Work out the finished part from the listing and answer in its coordinate system (mm). Round coordinates to 2 decimals unless told otherwise and drop trailing zeros. Write each loop counter-clockwise with the first axis right and the second up, starting at its lowest first coordinate (ties: lowest second). Pieces come first, ordered by that corner, then holes. Notation, with made-up numbers: (-0.75, 66) - (53.25, 66) arc R18 cw to (53.25, 97) - close; hole circle Ø5 at (0, -26.75). An arc over 180 degrees is marked (long way). Answer as a JSON object with one key per item and string values.
Autodesk Inventor part; units mm, degrees
ref_plane "YZ Plane" through (0, 0, 0) normal (1, 0, 0) x (0, 1, 0)
ref_plane "XZ Plane" through (0, 0, 0) normal (0, 1, 0) x (-1, 0, 0)
ref_plane "XY Plane" through (0, 0, 0) normal (0, 0, 1) x (1, 0, 0)
sketch "Sketch1" plane through (0, 0, 0) normal (0, 0, 1) x (1, 0, 0)
  line L0 (-262.5, 75) -> (262.5, 75)
  line L1 (262.5, 75) -> (262.5, 0)
  line L2 (262.5, 0) -> (-262.5, 0)
  line L3 (-262.5, 0) -> (-262.5, 75)
  line L4 (-262.5, 50) -> (-268.977, 50)
  line L5 (-268.977, 50) -> (-268.977, 25)
  line L6 (-268.977, 25) -> (-262.5, 25)
  line L7 (-262.5, 25) -> (-262.5, 50)
  line L8 (-212.5, 75) -> (-187.5, 75)
  line L9 (-187.5, 75) -> (-187.5, 81.477)
  line L10 (-187.5, 81.477) -> (-212.5, 81.477)
  line L11 (-212.5, 81.477) -> (-212.5, 75)
  line L12 (-12.5, 75) -> (12.5, 75)
  line L13 (12.5, 75) -> (12.5, 81.477)
  line L14 (12.5, 81.477) -> (-12.5, 81.477)
  line L15 (-12.5, 81.477) -> (-12.5, 75)
  point P0 (0, 0)
  point P1 (0, 0)
  point P2 (-268.977, 37.5)
  point P3 (-262.5, 37.5)
  point P4 (0, 81.477)
  point P5 (0, 75)
  dimension "d0" = 525
  dimension "d2" = 75
  dimension "d3" = 25
  dimension "d4" = 6.477
  dimension "d5" = 50
extrude "Extrusion1" add sketch "Sketch1" along normal blind 6.477
mirror "Mirror1" about plane through (0, 0, 0) normal (1, 0, 0) of "Extrusion1"
sketch "Sketch2" plane through (0, 0, 6.477) normal (0, 0, 1) x (1, 0, 0)
  line L0 (-187.5, 81.477) -> (-212.5, 81.477)
  line L1 (-262.5, 75) -> (-262.5, 50)
  line L2 (-268.977, 50) -> (-268.977, 25)
  line L3 (12.5, 81.477) -> (-12.5, 81.477)
  line L4 (-12.5, 75) -> (-187.5, 75)
  line L5 (-260, 39.5) -> (-258.5, 39.5)
  line L6 (-258.5, 39.5) -> (-258.5, 35.5)
  line L7 (-258.5, 35.5) -> (-260, 35.5)
  line L8 (-260, 35.5) -> (-260, 39.5)
  line L9 (-202, 72.5) -> (-198, 72.5)
  line L10 (-198, 72.5) -> (-198, 71)
  line L11 (-198, 71) -> (-202, 71)
  line L12 (-202, 71) -> (-202, 72.5)
  line L13 (-2, 72.5) -> (2, 72.5)
  line L14 (2, 72.5) -> (2, 71)
  line L15 (2, 71) -> (-2, 71)
  line L16 (-2, 71) -> (-2, 72.5)
  point P0 (0, 0)
  point P1 (-268.977, 37.5)
  point P2 (-260, 37.5)
  point P3 (-200, 72.5)
  point P4 (-200, 81.477)
  point P5 (0, 72.5)
  point P6 (0, 81.477)
  dimension "d8" = 4
  dimension "d10" = 1.5
  dimension "d11" = 2.5
  dimension "d13" = 2.5
extrude "Extrusion2" cut sketch "Sketch2" against normal through all
mirror "Mirror2" about plane through (0, 0, 0) normal (1, 0, 0) of "Extrusion2"
sketch "Sketch3" plane through (0, 0, 6.477) normal (0, 0, 1) x (1, 0, 0)
  line L0 (-262.5, 0) -> (262.5, 0)
  arc A0 (237.5, 0) -> (-237.5, 0) centre (0, -1872.7083) ccw
  point P0 (0, 0)
  point P1 (0, 15)
  point P2 (0, 0)
  dimension "d16" = 25
  dimension "d17" = 15
extrude "Extrusion3" cut sketch "Sketch3" against normal through all
properties part number "STRUT"
Item 1: A cutting plane is placed at B-B (y = 9.5). Write down the section's boundary in (x, z), and give its area (3 significant figures).
Results found:
{"outline": "(-262.5, 0) - (-143.99, 0) - (-143.99, 6.48) - (-262.5, 6.48) - close; (143.99, 0) - (262.5, 0) - (262.5, 6.48) - (143.99, 6.48) - close", "area": "1,540 mm²"}
Item 2: Each of these flat-tipped pins is pushed along its axis until it touches: P1, Ø5, axis at x = -89, y = 29.5, coming from the -Z side; P2, Ø1.9, axis at x = -235, z = 2, coming from the +Y side; P3, Ø1.2, axis at y = 72, z = 5, coming from the +X side; P4, Ø3, axis at y = 78, z = 1.5, coming from the -X side. Where does it stop, or does it pass through?
Results found:
{"P1": "z = 0", "P2": "y = 75", "P3": "x = 262.5", "P4": "x = -212.5"}
Item 3: A cutting plane is placed at A-A (z = 2.25). Give the number of separate pieces and of enclosed holes in the cut face, and give its area (3 significant figures).
Results found:
{"separate pieces": "1", "enclosed holes": "5", "area": "35,400 mm²"}
Item 4: A cutting plane is placed at D-D (x = -70.5). Write down the section's boundary in (y, z), and give its area (3 significant figures).
Results found:
{"outline": "(13.68, 0) - (75, 0) - (75, 6.48) - (13.68, 6.48) - close", "area": "397 mm²"}
Item 5: A cutting plane is placed at C-C (y = 63.5). Write down the section's boundary in (x, z), and give its area (3 significant figures).
Results found:
{"outline": "(-262.5, 0) - (262.5, 0) - (262.5, 6.48) - (-262.5, 6.48) - close", "area": "3,400 mm²"}
Item 6: Consider line 1 along Y through (x, z) = (9, 3.5); line 2 along X through (y, z) = (74, 4); line 3 along Y through (x, z) = (-201.5, 3.5). Determine where each line is inside the solid, lowest interval first.
Results found:
{"line 1": "14.98 to 81.48", "line 2": "-262.5 to 262.5", "line 3": "4.21 to 71, 72.5 to 81.48"}
Item 7: Determine the mould class of faces 1 (the cylindrical face through (3.334, 14.997, 3.284)), 2 (the flat face through (-4, 41, 6.477)) for opening direction X: pulls with the +X half, pulls with the -X half, needs draft (parallel to the pull), parting line crosses it, or undercut.
Results found:
{"face 1": "undercut", "face 2": "needs draft"}
